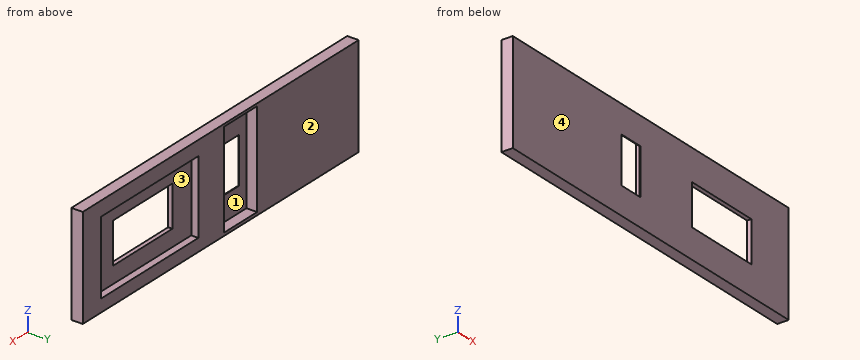
from build123d import *

# Parameters (mm, degrees)
SKETCH1_W           = 512.8
SKETCH1_H           = 142.48
BOSS_EXTRUDE1_DEPTH = 16
SKETCH5_W           = 180.81
SKETCH5_H           = 104.08
CUT_EXTRUDE2_DEPTH  = 10
SKETCH6_W           = 110.54
SKETCH6_H           = 57.54
CUT_EXTRUDE3_DEPTH  = 267.636306605
SKETCH7_W           = 61.93
SKETCH7_H           = 134.73
CUT_EXTRUDE4_DEPTH  = 15
SKETCH8_W           = 35
SKETCH8_H           = 65
CUT_EXTRUDE5_DEPTH  = 5


with BuildPart() as part:
    # Sketch1 → Boss-Extrude1 (new body)
    with BuildSketch(Plane(origin=(0, 0, 0), x_dir=(1, 0, 0), z_dir=(0, 1, 0))):
        with Locations((0, 0.16)):
            Rectangle(SKETCH1_W, SKETCH1_H)
    extrude(amount=BOSS_EXTRUDE1_DEPTH)

    # Sketch5 → Cut-Extrude2 (cut)
    with BuildSketch(Plane(origin=(0, 16, 0), x_dir=(1, 0, 0), z_dir=(0, 1, 0))):
        with Locations((131.895, 1.499952895)):
            Rectangle(SKETCH5_W, SKETCH5_H)
    extrude(amount=-CUT_EXTRUDE2_DEPTH, mode=Mode.SUBTRACT)

    # Sketch6 → Cut-Extrude3 (cut, through all)
    with BuildSketch(Plane(origin=(0, 16, 0), x_dir=(1, 0, 0), z_dir=(0, 1, 0))):
        with Locations((131.895, 1.429952895)):
            Rectangle(SKETCH6_W, SKETCH6_H)
    extrude(amount=-CUT_EXTRUDE3_DEPTH, mode=Mode.SUBTRACT)

    # Sketch7 → Cut-Extrude4 (cut)
    with BuildSketch(Plane(origin=(0, 16, 0), x_dir=(1, 0, 0), z_dir=(0, 1, 0))):
        with Locations((-36.795, -0.164973308)):
            Rectangle(SKETCH7_W, SKETCH7_H)
    extrude(amount=-CUT_EXTRUDE4_DEPTH, mode=Mode.SUBTRACT)

    # Sketch8 → Cut-Extrude5 (cut)
    with BuildSketch(Plane(origin=(0, 1, 0), x_dir=(1, 0, 0), z_dir=(0, 1, 0))):
        with Locations((-36.76, 0.349234115)):
            Rectangle(SKETCH8_W, SKETCH8_H)
    extrude(amount=-CUT_EXTRUDE5_DEPTH, mode=Mode.SUBTRACT)


solid = part.part
Verification items for the finished model (mm, model axes). Face numbers are marked on the shaded views. A direction names the side the tool comes from. Coordinates: 2 decimals unless noted, no trailing zeros. Order: outer loops, then holes, each group sorted by start corner. A loop starts at its lowest first (then second) coordinate and runs counter-clockwise, first axis right, second up. Notation, with made-up numbers: M 60.5,72.5 L 68.5,72.5 A15 ccw 68.5,81.5 Z; hole C 14.25,10 d1. An arc over 180 degrees is marked long. One line per item, written item: value. Start each with the question number.
Item 1: Depth check by flat-ended pin: P1, Ø3, axis at x = -58.5, z = 44, coming from the +Y side. Enter the tip coordinate at first touch or a pass-through.
Item 2: Sectioned sample at C-C on y = 11.75. Record the cut outline in (x, z), then the cut area to 3 significant figures.
Item 3: Thickness scan on probe 1 along X at (y, z) = (2.75, 18.5) (3 decimals); probe 2 along X at (y, z) = (12, 48.5); probe 3 along Z at (x, y) = (98.5, 14.75). Record the ranges inside material, lowest first.
Item 4: Mould release check, pull along Z, two halves, no side actions. Record for the marked faces 1 and 2: pulls with the +Z half, pulls with the -Z half, needs draft (parallel to the pull), parting line crosses it, or undercut.
Item 5: Sectioned sample at A-A on z = 6. Record the cut outline in (x, y) (3 decimals), then the cut area to 3 significant figures.
Item 6: Sectioned sample at B-B on x = 136. Record the cut outline in (y, z), then the cut area to 3 significant figures.
Item 7: Access from +Z, -Z, +X, -X, +Y, -Y to the whole of each face (thin tool, end or side, straight path). Record for the marked faces 3 and 4.
Item 8: Sectioned sample at D-D on z = 42. Record the cut outline in (x, y).
Calculated:
1. P1: y = 1
2. outline: M -256.4,-71.4 L 256.4,-71.4 L 256.4,71.08 L -256.4,71.08 Z; hole M -67.76,-67.2 L -5.83,-67.2 L -5.83,67.53 L -67.76,67.53 Z; hole M 41.49,-53.54 L 222.3,-53.54 L 222.3,50.54 L 41.49,50.54 Z
2. area: 45,900 mm^2
3. probe 1: -256.4 to -67.76, -5.83 to 76.625, 187.165 to 256.4
3. probe 2: -256.4 to -67.76, -5.83 to 41.49, 222.3 to 256.4
3. probe 3: -71.4 to -53.54, 50.54 to 71.08
4. face 1: undercut
4. face 2: needs draft
5. outline: M -256.4,0 L -54.26,0 L -54.26,1 L -67.76,1 L -67.76,16 L -256.4,16 Z; M -19.26,0 L 76.625,0 L 76.625,6 L 41.49,6 L 41.49,16 L -5.83,16 L -5.83,1 L -19.26,1 Z; M 187.165,0 L 256.4,0 L 256.4,16 L 222.3,16 L 222.3,6 L 187.165,6 Z
5. area: 4,770 mm^2
6. outline: M 0,-71.4 L 16,-71.4 L 16,-53.54 L 6,-53.54 L 6,-30.2 L 0,-30.2 Z; M 0,27.34 L 6,27.34 L 6,50.54 L 16,50.54 L 16,71.08 L 0,71.08 Z
6. area: 894 mm^2
7. face 3: +Y
7. face 4: +Z, -Z, +X, -X, -Y
8. outline: M -256.4,0 L 256.4,0 L 256.4,16 L 222.3,16 L 222.3,6 L 41.49,6 L 41.49,16 L -5.83,16 L -5.83,1 L -67.76,1 L -67.76,16 L -256.4,16 Z
